```python
from build123d import *

# Parameters (mm, degrees)
F1_DEPTH = 1
F3_DEPTH = 3


with BuildPart() as f1:
    # F0 (on Front) → F1 (new body)
    with BuildSketch(Plane.XZ):
        with BuildLine():
            Line((14.090503, 21.313837), (35, 21.313837))
            Line((35, 21.313837), (35, 44.340667))
            ThreePointArc((35, 44.340667), (0, 56.489775), (-35, 44.340667))
            Line((-35, 44.340667), (-35, 21.313837))
            Line((-35, 21.313837), (-14.090503, 21.313837))
            ThreePointArc((-14.090503, 21.313837), (0, 25.55038), (14.090503, 21.313837))
        make_face()
    extrude(amount=-F1_DEPTH)

    # F2 (on face) → F3 (join)
    with BuildSketch(Plane(origin=(0, 1, 0), x_dir=(-1, 0, 0), z_dir=(0, 1, 0))):
        with BuildLine():
            ThreePointArc((33.5, 43.607628), (-1e-06, 54.989774), (-33.500001, 43.607627))
            Line((-33.500001, 43.607627), (-33.500001, 22.813837))
            Line((-33.500001, 22.813837), (-14.534507, 22.813837))
            ThreePointArc((-14.534507, 22.813837), (0, 27.05038), (14.534507, 22.813837))
            Line((14.534507, 22.813837), (33.5, 22.813837))
            Line((33.5, 22.813837), (33.5, 43.607628))
        make_face()
    extrude(amount=F3_DEPTH)


solid = f1.part
```
Part model, mm, in its own coordinate system. A direction names the side the tool comes from. Round coordinates to 2 decimals unless told otherwise and drop trailing zeros. Order: outer loops, then holes, each group sorted by start corner. A loop starts at its lowest first (then second) coordinate and runs counter-clockwise, first axis right, second up. Notation, with made-up numbers: M -32.75,7.25 L 7.25,7.25 A27 ccw 7.25,23.25 Z; hole C 43.25,-38.5 d9. An arc over 180 degrees is marked long. Put each result on its own line as item: value. Start each with the question number.
1. Slice it at A-A on z = 39. List the corners of the cut face in (x, y).
2. Two-plate mould, pull along X, no slides. Class faces 6 (the face through (0, 1, 26)), 7 (the face through (-0.504, 2.479, 54.987)), 8 (the face through (-0.21, 0.49, 25.55)), 9 (the face through (33.5, 2, 33)): +X half, -X half, draft (parallel to the pull), parting line (faces both ways), or undercut.
3. Slice it at C-C on y = 2.2. List the corners of the cut face in (x, z).
4. Tool access for faces 1 (the face through (0.528, 0.493, 56.487)), 2 (the face through (24, 2, 22.814)), 3 (the face through (0, 0, 39)), 4 (the face through (-33.5, 2, 33)), 5 (the face through (0.21, 2.48, 27.05)): list every direction of +Z, -Z, +X, -X, +Y, -Y with a clear straight run to the whole face (end or side of a thin tool).
5. Slice it at B-B on x = 0. List the corners of the cut face in (y, z).
6. Drop a flat-ended pin along its axis: pin 1 (0.9 mm diameter, centred on x = -26.5, y = 2.5, fed in from -Z). Give the stop position or say it passes through.
7. Drill centre lines: probe 1 along X at (y, z) = (3.5, 43); probe 2 along X at (y, z) = (1.2, 25); probe 3 along Z at (x, y) = (-27.5, 2.85). Where is each one in solid material? Low to high. Write a range as [from, to].
Findings:
1. outline: M -35,0 L 35,0 L 35,1 L 33.5,1 L 33.5,4 L -33.5,4 L -33.5,1 L -35,1 Z
2. face 6: undercut
2. face 7: parting line
2. face 8: undercut
2. face 9: +X half
3. outline: M -33.5,22.81 L -14.53,22.81 A27.05 cw 14.53,22.81 L 33.5,22.81 L 33.5,43.61 A54.99 ccw -33.5,43.61 Z
4. face 1: +Z, +Y, -Y
4. face 2: -Z, +X, -X, +Y
4. face 3: +Z, -Z, +X, -X, -Y
4. face 4: +Z, -Z, -X, +Y
4. face 5: -Z, +Y
5. outline: M 0,25.55 L 1,25.55 L 1,27.05 L 4,27.05 L 4,54.99 L 1,54.99 L 1,56.49 L 0,56.49 Z
6. pin 1: z = 22.81
7. probe 1: [-33.5, 33.5]
7. probe 2: [-33.5, -10.33], [10.33, 33.5]
7. probe 3: [22.81, 47.62]
